Autodesk Fusion 360 part; units mm, degrees
sketch "Skizze1" plane through (0, 0, 0) normal (0, 0, 1) x (1, 0, 0)
  circle A0 centre (-25, -56.5195) radius 2.05
  circle A1 centre (-25, -93.5195) radius 2.05
  circle A2 centre (-25, -75.0195) radius 4.5
  circle A3 centre (25, -93.5195) radius 2.05
  circle A4 centre (25, -56.5195) radius 2.05
  circle A5 centre (25, -75.0195) radius 4.5
  line L0 (40, -100.0195) -> (-40, -100.0195)
  line L1 (-55, -85.0195) -> (-55, -35.0195)
  line L2 (-70, -20.0195) -> (-85, -20.0195)
  line L3 (-100, -5.0195) -> (-100, 134.9805)
  line L4 (-85, 149.9805) -> (85, 149.9805)
  line L5 (100, 134.9805) -> (100, -5.0195)
  line L6 (85, -20.0195) -> (70, -20.0195)
  line L7 (55, -35.0195) -> (55, -85.0195)
  line L8 (70, 129.9805) -> (-70, 129.9805)
  line L9 (-80, 119.9805) -> (-80, 99.9805)
  line L10 (-70, 89.9805) -> (70, 89.9805)
  line L11 (80, 99.9805) -> (80, 119.9805)
  line L12 (9.75, -0.0695) -> (40.25, -0.0695)
  line L13 (40.25, 66.4305) -> (9.75, 66.4305)
  circle A6 centre (34, 70.6805) radius 2.05
  circle A7 centre (34, -4.3195) radius 2.05
  line L14 (40.25, -0.0695) -> (40.25, 66.4305)
  circle A8 centre (16, -4.3195) radius 2.05
  line L15 (9.75, 66.4305) -> (9.75, -0.0695)
  circle A9 centre (16, 70.6805) radius 2.05
  line L16 (-40.25, -0.0695) -> (-9.75, -0.0695)
  line L17 (-9.75, 66.4305) -> (-40.25, 66.4305)
  circle A10 centre (-16, 70.6805) radius 2.05
  circle A11 centre (-16, -4.3195) radius 2.05
  line L18 (-9.75, -0.0695) -> (-9.75, 66.4305)
  circle A12 centre (-34, -4.3195) radius 2.05
  line L19 (-40.25, 66.4305) -> (-40.25, -0.0695)
  circle A13 centre (-34, 70.6805) radius 2.05
  arc A14 (100, 134.9805) -> (85, 149.9805) centre (85, 134.9805) ccw
  arc A15 (-85, 149.9805) -> (-100, 134.9805) centre (-85, 134.9805) ccw
  arc A16 (-100, -5.0195) -> (-85, -20.0195) centre (-85, -5.0195) ccw
  arc A17 (85, -20.0195) -> (100, -5.0195) centre (85, -5.0195) ccw
  arc A18 (40, -100.0195) -> (55, -85.0195) centre (40, -85.0195) ccw
  arc A19 (-55, -85.0195) -> (-40, -100.0195) centre (-40, -85.0195) ccw
  arc A20 (-55, -35.0195) -> (-70, -20.0195) centre (-70, -35.0195) ccw
  arc A21 (70, -20.0195) -> (55, -35.0195) centre (70, -35.0195) ccw
  line L20 (-75, 59.9805) -> (-65, 59.9805)
  line L21 (-60, 54.9805) -> (-60, 4.9805)
  line L22 (-65, -0.0195) -> (-75, -0.0195)
  line L23 (-80, 4.9805) -> (-80, 54.9805)
  arc A22 (-80, 99.9805) -> (-70, 89.9805) centre (-70, 99.9805) ccw
  arc A23 (-70, 129.9805) -> (-80, 119.9805) centre (-70, 119.9805) ccw
  arc A24 (70, 89.9805) -> (80, 99.9805) centre (70, 99.9805) ccw
  arc A25 (80, 119.9805) -> (70, 129.9805) centre (70, 119.9805) ccw
  arc A26 (-60, 54.9805) -> (-65, 59.9805) centre (-65, 54.9805) ccw
  arc A27 (-75, 59.9805) -> (-80, 54.9805) centre (-75, 54.9805) ccw
  arc A28 (-80, 4.9805) -> (-75, -0.0195) centre (-75, 4.9805) ccw
  arc A29 (-65, -0.0195) -> (-60, 4.9805) centre (-65, 4.9805) ccw
  line L24 (75, 59.9805) -> (65, 59.9805)
  line L25 (60, 54.9805) -> (60, 4.9805)
  line L26 (65, -0.0195) -> (75, -0.0195)
  line L27 (80, 4.9805) -> (80, 54.9805)
  arc A30 (80, 54.9805) -> (75, 59.9805) centre (75, 54.9805) ccw
  arc A31 (65, 59.9805) -> (60, 54.9805) centre (65, 54.9805) ccw
  arc A32 (60, 4.9805) -> (65, -0.0195) centre (65, 4.9805) ccw
  arc A33 (75, -0.0195) -> (80, 4.9805) centre (75, 4.9805) ccw
  circle A34 centre (90, 69.9805) radius 3.05
  circle A35 centre (-90, 69.9805) radius 3.05
  circle A36 centre (90, 139.9805) radius 3.05
  circle A37 centre (-90, 139.9805) radius 3.05
  circle A38 centre (90, -10) radius 3.05
  circle A39 centre (-90, -10) radius 3.05
  circle A40 centre (0, 69.9805) radius 3.05
  circle A41 centre (0, -90.0195) radius 3.05
  circle A42 centre (0, -10) radius 3.05
  dimension "d5" = 9
  dimension "d6" = 4.1
  dimension "d7" = 18.5
  dimension "d8" = 4.1
  dimension "d9" = 18.5
  dimension "d10" = 9
  dimension "d11" = 4.1
  dimension "d12" = 18.5
  dimension "d13" = 4.1
  dimension "d14" = 18.5
  dimension "d15" = 25
  dimension "d16" = 200
  dimension "d18" = 25
  dimension "d47" = 25
  dimension "d68" = 15.25
  dimension "d69" = 15.25
  dimension "d70" = 33.25
  dimension "d71" = 33.25
  dimension "d72" = 4.1
  dimension "d73" = 18
  dimension "d74" = 75
  dimension "d78" = 15.25
  dimension "d79" = 15.25
  dimension "d80" = 15.25
  dimension "d81" = 33.25
  dimension "d82" = 33.25
  dimension "d83" = 4.1
  dimension "d84" = 18
  dimension "d85" = 75
  dimension "d89" = 15.25
  dimension "d90" = 9
  dimension "d91" = 37.5
  dimension "d94" = 25
  dimension "d95" = 25
  dimension "d98" = 37.5
  dimension "d99" = 9
  dimension "d100" = 15
  dimension "d101" = 15
  dimension "d104" = 20
  dimension "d105" = 20
  dimension "d106" = 20
  dimension "d107" = 40
  dimension "d108" = 10
  dimension "d109" = 5
  dimension "d110" = 5
  dimension "d113" = 55
  dimension "d114" = 55
  dimension "d115" = 250
  dimension "d116" = 170
  dimension "d117" = 20
  dimension "d118" = 20
  dimension "d120" = 20
  dimension "d121" = 60
  dimension "d122" = 170
  dimension "d123" = 20
  dimension "d124" = 20
  dimension "d125" = 60
  dimension "d126" = 20
  dimension "d127" = 6.1
  dimension "d128" = 10
  dimension "d129" = 10
  dimension "d130" = 10
  dimension "d131" = 10
  dimension "d132" = 10
  dimension "d133" = 10
  dimension "d134" = 10
  dimension "d135" = 10
  dimension "d136" = 10
  dimension "d137" = 10
  dimension "d139" = 100
  dimension "d194" = 18.2
  dimension "d195" = 18.2
  dimension "d197" = 90
  dimension "d198" = 90
extrude "Extrusion3" add sketch "Skizze1" along normal blind 10
sketch "Skizze2" plane through (0, 0, 10) normal (0, 0, 1) x (1, 0, 0)
  circle A0 centre (-90, 69.9805) radius 3.05
  circle A1 centre (0, -90.0195) radius 3.05
  circle A2 centre (0, -10) radius 3.05
  circle A3 centre (0, 69.9805) radius 3.05
  circle A4 centre (-90, -10) radius 3.05
  circle A5 centre (90, -10) radius 3.05
  circle A6 centre (-90, 139.9805) radius 3.05
  circle A7 centre (90, 139.9805) radius 3.05
  circle A8 centre (-25, -93.5195) radius 2.05
  circle A9 centre (-25, -75.0195) radius 4.5
  circle A10 centre (25, -93.5195) radius 2.05
  circle A11 centre (16, 70.6805) radius 2.05
  circle A12 centre (-16, 70.6805) radius 2.05
  arc A13 (75, -0.0195) -> (80, 4.9805) centre (75, 4.9805) ccw
  line L0 (75, -0.0195) -> (65, -0.0195)
  arc A14 (60, 4.9805) -> (65, -0.0195) centre (65, 4.9805) ccw
  line L1 (60, 4.9805) -> (60, 54.9805)
  arc A15 (65, 59.9805) -> (60, 54.9805) centre (65, 54.9805) ccw
  line L2 (65, 59.9805) -> (75, 59.9805)
  arc A16 (80, 54.9805) -> (75, 59.9805) centre (75, 54.9805) ccw
  line L3 (80, 54.9805) -> (80, 4.9805)
  circle A17 centre (-16, -4.3195) radius 2.05
  circle A18 centre (90, 69.9805) radius 3.05
  circle A19 centre (-25, -56.5195) radius 2.05
  circle A20 centre (-34, 70.6805) radius 2.05
  line L4 (-40.25, -0.0695) -> (-40.25, 66.4305)
  line L5 (-40.25, 66.4305) -> (-9.75, 66.4305)
  line L6 (-9.75, 66.4305) -> (-9.75, -0.0695)
  line L7 (-9.75, -0.0695) -> (-40.25, -0.0695)
  circle A21 centre (-34, -4.3195) radius 2.05
  arc A22 (-80, 4.9805) -> (-75, -0.0195) centre (-75, 4.9805) ccw
  line L8 (-80, 4.9805) -> (-80, 54.9805)
  arc A23 (-75, 59.9805) -> (-80, 54.9805) centre (-75, 54.9805) ccw
  line L9 (-75, 59.9805) -> (-65, 59.9805)
  arc A24 (-60, 54.9805) -> (-65, 59.9805) centre (-65, 54.9805) ccw
  line L10 (-60, 54.9805) -> (-60, 4.9805)
  arc A25 (-65, -0.0195) -> (-60, 4.9805) centre (-65, 4.9805) ccw
  line L11 (-65, -0.0195) -> (-75, -0.0195)
  arc A26 (80, 119.9805) -> (70, 129.9805) centre (70, 119.9805) ccw
  line L12 (80, 119.9805) -> (80, 99.9805)
  arc A27 (70, 89.9805) -> (80, 99.9805) centre (70, 99.9805) ccw
  line L13 (70, 89.9805) -> (-70, 89.9805)
  arc A28 (-80, 99.9805) -> (-70, 89.9805) centre (-70, 99.9805) ccw
  line L14 (-80, 99.9805) -> (-80, 119.9805)
  arc A29 (-70, 129.9805) -> (-80, 119.9805) centre (-70, 119.9805) ccw
  line L15 (-70, 129.9805) -> (70, 129.9805)
  circle A30 centre (34, 70.6805) radius 2.05
  circle A31 centre (25, -56.5195) radius 2.05
  circle A32 centre (16, -4.3195) radius 2.05
  circle A33 centre (25, -75.0195) radius 4.5
  circle A34 centre (34, -4.3195) radius 2.05
  line L16 (9.75, -0.0695) -> (9.75, 66.4305)
  line L17 (9.75, 66.4305) -> (40.25, 66.4305)
  line L18 (40.25, 66.4305) -> (40.25, -0.0695)
  line L19 (40.25, -0.0695) -> (9.75, -0.0695)
  arc A35 (85, -20.0195) -> (100, -5.0195) centre (85, -5.0195) ccw
  line L20 (100, -5.0195) -> (100, 134.9805)
  arc A36 (100, 134.9805) -> (85, 149.9805) centre (85, 134.9805) ccw
  line L21 (85, 149.9805) -> (-85, 149.9805)
  arc A37 (-85, 149.9805) -> (-100, 134.9805) centre (-85, 134.9805) ccw
  line L22 (-100, 134.9805) -> (-100, -5.0195)
  arc A38 (-100, -5.0195) -> (-85, -20.0195) centre (-85, -5.0195) ccw
  line L23 (-85, -20.0195) -> (-70, -20.0195)
  arc A39 (-55, -35.0195) -> (-70, -20.0195) centre (-70, -35.0195) ccw
  line L24 (-55, -35.0195) -> (-55, -85.0195)
  arc A40 (-55, -85.0195) -> (-40, -100.0195) centre (-40, -85.0195) ccw
  line L25 (-40, -100.0195) -> (40, -100.0195)
  arc A41 (40, -100.0195) -> (55, -85.0195) centre (40, -85.0195) ccw
  line L26 (55, -85.0195) -> (55, -35.0195)
  arc A42 (70, -20.0195) -> (55, -35.0195) centre (70, -35.0195) ccw
  line L27 (70, -20.0195) -> (85, -20.0195)
  line L28 (85, -20.0195) -> (70, -20.0195)
  line L29 (100, 134.9805) -> (100, -5.0195)
  line L30 (-70, -20.0195) -> (-85, -20.0195)
  line L31 (-100, -5.0195) -> (-100, 134.9805)
  line L32 (60, 54.9805) -> (60, 4.9805)
  line L33 (-60, 54.9805) -> (-60, 4.9805)
  line L34 (-48.25, 56.4305) -> (-46.25, 56.4305)
  line L35 (-45.75, 55.9305) -> (-45.75, 53.9305)
  line L36 (-46.25, 53.4305) -> (-48.25, 53.4305)
  line L37 (-48.75, 53.9305) -> (-48.75, 55.9305)
  arc A43 (-48.25, 56.4305) -> (-48.75, 55.9305) centre (-48.25, 55.9305) ccw
  arc A44 (-45.75, 55.9305) -> (-46.25, 56.4305) centre (-46.25, 55.9305) ccw
  arc A45 (-46.25, 53.4305) -> (-45.75, 53.9305) centre (-46.25, 53.9305) ccw
  arc A46 (-48.75, 53.9305) -> (-48.25, 53.4305) centre (-48.25, 53.9305) ccw
  line L38 (-40.25, 66.4305) -> (-40.25, -0.0695)
  line L39 (-9.75, 66.4305) -> (-40.25, 66.4305)
  line L40 (48.75, 55.9305) -> (48.75, 53.9305)
  arc A47 (46.25, 56.4305) -> (45.75, 55.9305) centre (46.25, 55.9305) ccw
  arc A48 (48.25, 53.4305) -> (48.75, 53.9305) centre (48.25, 53.9305) ccw
  arc A49 (45.75, 53.9305) -> (46.25, 53.4305) centre (46.25, 53.9305) ccw
  line L41 (48.25, 53.4305) -> (46.25, 53.4305)
  line L42 (46.25, 56.4305) -> (48.25, 56.4305)
  line L43 (45.75, 53.9305) -> (45.75, 55.9305)
  arc A50 (48.75, 55.9305) -> (48.25, 56.4305) centre (48.25, 55.9305) ccw
  line L44 (40.25, -0.0695) -> (40.25, 66.4305)
  line L45 (40.25, 66.4305) -> (9.75, 66.4305)
  line L46 (1.75, 55.9305) -> (1.75, 53.9305)
  arc A51 (-0.75, 56.4305) -> (-1.25, 55.9305) centre (-0.75, 55.9305) ccw
  arc A52 (1.25, 53.4305) -> (1.75, 53.9305) centre (1.25, 53.9305) ccw
  arc A53 (-1.25, 53.9305) -> (-0.75, 53.4305) centre (-0.75, 53.9305) ccw
  line L47 (1.25, 53.4305) -> (-0.75, 53.4305)
  line L48 (-0.75, 56.4305) -> (1.25, 56.4305)
  line L49 (-1.25, 53.9305) -> (-1.25, 55.9305)
  arc A54 (1.75, 55.9305) -> (1.25, 56.4305) centre (1.25, 55.9305) ccw
  line L50 (9.75, 66.4305) -> (9.75, -0.0695)
  point P0 (-20, 0)
  point P1 (-20, 0)
  dimension "d177" = 3
  dimension "d178" = 3
  dimension "d179" = 0.5
  dimension "d180" = 5.5
  dimension "d181" = 10
  dimension "d182" = 3
  dimension "d183" = 3
  dimension "d184" = 0.5
  dimension "d185" = 5.5
  dimension "d186" = 10
  dimension "d187" = 3
  dimension "d188" = 3
  dimension "d189" = 0.5
  dimension "d190" = 8
  dimension "d191" = 10
extrude "Extrusion5" cut sketch "Skizze2" against normal blind 10 contours L34 L35 L36 L37 A43 A44 A45 A46 | L40 A47 A48 A49 L41 L42 L43 A50 | L46 A51 A52 A53 L47 L48 L49 A54
equation "d68 = 15 mm + tolerance"
equation "d69 = 15 mm + tolerance"
equation "d70 = 33 mm + tolerance"
equation "d71 = 33 mm + tolerance"
equation "d78 = 15 mm + tolerance"
equation "d79 = 15 mm + tolerance"
equation "d80 = 15 mm + tolerance"
equation "d81 = 33 mm + tolerance"
equation "d82 = 33 mm + tolerance"
equation "d89 = 15 mm + tolerance"
equation "tolerance = 0.25 mm"
For this review, take the finished solid that the model builds, in its own axes (mm). A direction names the side the tool comes from. Give positions to 0.01 mm unless a question says otherwise; leave off trailing zeros. Loops run counter-clockwise (first coordinate to the right, second up) from the corner with the lowest first, then second, coordinate; pieces in that order, holes last. Notation, with made-up numbers: M 29.25,-17 L 77.25,-17 A14 ccw 77.25,-6 Z; hole C -29.75,72 d5. An arc over 180 degrees is marked long. One line per item, written item: value. Start each with the question number.
Q1. Draft analysis for pull direction X (two halves, no side actions). For faces 1 (the face through (-1, 27, 0)), 2 (the face through (100, 66, 5)), 3 (the face through (-92.42, 141.84, 4.93)), 4 (the face through (24.024, -70.627, 4.93)), state which applies: released by +X, released by -X, zero draft, split by the parting line, or undercut.
Q2. Add section A-A (y = 41.5). Give the boundary of the cut face in (x, z).
Q3. Clearance check with flat-ended pins moving along their axes: pin 1 Ø3.5 at (x, y) = (34, 70.68) entering from -Z; pin 2 Ø3 at (x, z) = (79.5, 3.5) entering from -Y. State where each tip first meets the part, or that it passes through.
Q4. Add section C-C (x = 6). Give the boundary of the cut face in (y, z), and give its area (3 significant figures).
Q5. Add section B-B (y = 111.5). Give the boundary of the cut face in (x, z).
Q6. Machinability: for faces 5 (the face through (1, -100.02, 5)), 6 (the face through (-40.25, 34, 5)), 7 (the face through (78, -20.02, 5)), which of the approach directions +Z, -Z, +X, -X, +Y, -Y give a long, thin tool a straight path to every point of the face, cutting with its end or side? Answer none if there is none.
Q7. Add section D-D (z = 5.25). Count the separate pieces of the cut face and the enclosed holes in it, and give its area (3 significant figures).
Q8. For L1, parallel to Y at x = 0, z = 8.25; L2, parallel to Y at x = -20, z = 2; L3, parallel to Y at x = -25, z = 7.5, list the stretches that pass through material, from the lowest coordinate up.
Reply:
1. face 1: zero draft
1. face 2: released by +X
1. face 3: undercut
1. face 4: undercut
2. outline: M -100,0 L -80,0 L -80,10 L -100,10 Z; M -60,0 L -40.25,0 L -40.25,10 L -60,10 Z; M -9.75,0 L 9.75,0 L 9.75,10 L -9.75,10 Z; M 40.25,0 L 60,0 L 60,10 L 40.25,10 Z; M 80,0 L 100,0 L 100,10 L 80,10 Z
3. pin 1: through
3. pin 2: y = -20.02
4. outline: M -100.02,0 L 89.98,0 L 89.98,10 L -100.02,10 Z; M 129.98,0 L 149.98,0 L 149.98,10 L 129.98,10 Z
4. area: 2,100 mm²
5. outline: M -100,0 L -80,0 L -80,10 L -100,10 Z; M 80,0 L 100,0 L 100,10 L 80,10 Z
6. face 5: +Z, -Z, +X, -X, -Y
6. face 6: +Z, -Z
6. face 7: +Z, -Z, +X, -Y
7. separate pieces: 1
7. enclosed holes: 31
7. area: 29,300 mm²
8. L1: -100.02 to -93.07, -86.97 to -13.05, -6.95 to 53.43, 56.43 to 66.93, 73.03 to 89.98, 129.98 to 149.98
8. L2: -100.02 to -0.07, 66.43 to 89.98, 129.98 to 149.98
8. L3: -100.02 to -95.57, -91.47 to -79.52, -70.52 to -58.57, -54.47 to -0.07, 66.43 to 89.98, 129.98 to 149.98
